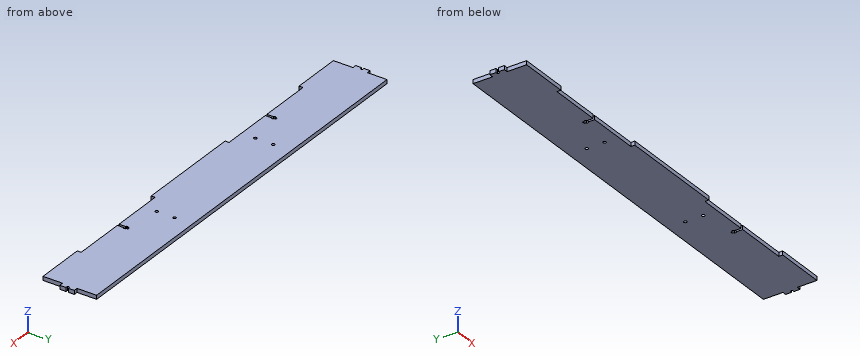
from build123d import *

# Parameters (mm, degrees)
BOSS_EXTRUDE1_DEPTH = 5.5
SKETCH2_R           = 2.1
CUT_EXTRUDE1_DEPTH  = 907.379197687


with BuildPart() as part:
    # Sketch1 → Boss-Extrude1 (new body)
    with BuildSketch(Plane.XY):
        Polygon((308.5, 78), (308.5, 50.625), (303, 50.625), (303, 42.125), (306.25, 42.125), (306.25, 40.5), (306.25, 38.875), (303, 38.875), (303, 30.375), (308.5, 30.375), (308.5, 3), (378, 3), (378, 8.5), (451.375, 8.5), (451.375, 17.95), (450.125, 17.95), (450.125, 20.6), (451.375, 20.6), (451.375, 23.25), (454.625, 23.25), (454.625, 20.6), (455.875, 20.6), (455.875, 17.95), (454.625, 17.95), (454.625, 8.5), (528, 8.5), (528, 3), (678, 3), (678, 8.5), (751.375, 8.5), (751.375, 17.95), (750.125, 17.95), (750.125, 20.6), (751.375, 20.6), (751.375, 23.25), (754.625, 23.25), (754.625, 20.6), (755.875, 20.6), (755.875, 17.95), (754.625, 17.95), (754.625, 8.5), (828, 8.5), (828, 3), (897.5, 3), (897.5, 30.375), (903, 30.375), (903, 38.875), (899.75, 38.875), (899.75, 40.5), (899.75, 42.125), (903, 42.125), (903, 50.625), (897.5, 50.625), (897.5, 78), align=None)
    extrude(amount=BOSS_EXTRUDE1_DEPTH)

    # Sketch2 → Cut-Extrude1 (cut, through all)
    with BuildSketch(Plane.XY.offset(5.5)):
        with Locations((503, 53)):
            Circle(SKETCH2_R)
        with Locations((503, 28)):
            Circle(SKETCH2_R)
        with Locations((703, 28)):
            Circle(SKETCH2_R)
        with Locations((703, 53)):
            Circle(SKETCH2_R)
    extrude(amount=-CUT_EXTRUDE1_DEPTH, mode=Mode.SUBTRACT)


solid = part.part
Could you check a few things on this model? Use its own coordinates, in mm. Round coordinates to 2 decimals unless told otherwise and drop trailing zeros. Loops run counter-clockwise (first coordinate to the right, second up) from the corner with the lowest first, then second, coordinate; pieces in that order, holes last. Notation, with made-up numbers: (-26, 52) - (25, 52) arc R17 cw to (25, 67) - close; hole circle Ø9 at (17, 37.25). An arc over 180 degrees is marked (long way). Write item = value, one per line.
1) Imagine slicing it at C-C (y = 70.5). Please give me the cut outline in (x, z).
Computed:
outline = (308.5, 0) - (897.5, 0) - (897.5, 5.5) - (308.5, 5.5) - close
2) Imagine slicing it at A-A (z = 2.35). Give the number of separate pieces and of enclosed holes in the cut face, and give its area (3 significant figures).
Computed:
separate_pieces = 1
enclosed_holes = 4
area = 42,600 mm2
3) Imagine slicing it at B-B (x = 710.5). Please give me the cut outline in (y, z).
Computed:
outline = (8.5, 0) - (78, 0) - (78, 5.5) - (8.5, 5.5) - close
4) I need wall thicknesses on line 1 along Y through (x, z) = (503, 1.5); line 2 along X through (y, z) = (18, 2.65) (3 decimals); line 3 along Y through (x, z) = (755.5, 2.2). Which ranges of each line are inside material? Lowest first, please. Write a range as from..to.
Computed:
line_1 = 8.5..25.9, 30.1..50.9, 55.1..78
line_2 = 308.5..450.125, 455.875..750.125, 755.875..897.5
line_3 = 8.5..17.95, 20.6..78
5) I'm going to push flat-ended pins straight in: P1, Ø1.4, axis at x = 455.5, z = 3.5, coming from the -Y side; P2, Ø3, axis at y = 22, z = 1.5, coming from the -X side; P3, Ø2.5, axis at x = 304.5, z = 2, coming from the +Y side (3 decimals). Where does each tip first touch, or does it pass through?
Computed:
P1 = 8.5
P2 = 308.5
P3 = 50.625
